from build123d import *

# Parameters (mm, degrees)
F0_W     = 93.609646
F0_H     = 82.611128
F1_DEPTH = 45.649247
F2_SIZE  = 1.27
F3_R     = 12.7


with BuildPart() as f1:
    # F0 (on Top) → F1 (new body)
    with BuildSketch(Plane.XY):
        with Locations((3.299557, -1.955293)):
            Rectangle(F0_W, F0_H)
    extrude(amount=F1_DEPTH)

    # F2
    f2_edges = [f1.edges().sort_by_distance(p)[0] for p in [
        (-43.505266, -43.260857, 22.824624),
        (50.10438, -43.260857, 22.824624),
        (3.299557, -43.260857, 0),
        (3.299557, -43.260857, 45.649247),
    ]]
    chamfer(f2_edges, length=F2_SIZE)

    # F3
    f3_edges = [f1.edges().sort_by_distance(p)[0] for p in [
        (50.10438, 39.350271, 22.824624),
        (-43.505266, 39.350271, 22.824624),
        (3.299557, 39.350271, 0),
        (3.299557, 39.350271, 45.649247),
    ]]
    fillet(f3_edges, radius=F3_R)


solid = f1.part
Could you check a few things on this model? Use its own coordinates, in mm. Give positions to 0.01 mm unless a question says otherwise; leave off trailing zeros. Write each loop counter-clockwise with the first axis right and the second up, starting at its lowest first coordinate (ties: lowest second). Pieces come first, ordered by that corner, then holes. Notation, with made-up numbers: (50, 82.5) -> (71, 82.5) arc R27 cw to (71, 113.5) -> close; hole circle Ø3 at (-39, -18.75). An arc over 180 degrees is marked (long way). Answer as a JSON object with one key per item and string values.
Q1. Suppose I cut it at C-C on y = 31. Write out the boundary of the cut face in (x, z), then the cut area to 3 significant figures.
Taken from the geometry:
{"outline": "(-42.74, 0.77) -> (49.34, 0.77) -> (49.34, 44.88) -> (-42.74, 44.88) -> close", "area": "4,060 mm²"}
Q2. Suppose I cut it at B-B on z = 3.5. Write out the boundary of the cut face in (x, y).
Taken from the geometry:
{"outline": "(-43.51, -41.99) -> (-42.24, -43.26) -> (48.83, -43.26) -> (50.1, -41.99) -> (50.1, 26.65) arc R12.7 ccw to (46.6, 35.41) -> (-40.01, 35.41) arc R12.7 ccw to (-43.51, 26.65) -> close"}
Q3. Please list where these lines run through material, in increasing order: L1, parallel to Y at x = -7.5, z = 6; L2, parallel to Y at x = -31, z = 29; L3, parallel to X at y = 28.5, z = 17.
Taken from the geometry:
{"L1": "y = -43.26 to 37.44", "L2": "y = -43.26 to 39.35", "L3": "x = -43.37 to 49.97"}
Q4. Suppose I cut it at A-A on x = 21. Write out the boundary of the cut face in (y, z), then the cut area to 3 significant figures.
Taken from the geometry:
{"outline": "(-43.26, 1.27) -> (-41.99, 0) -> (26.65, 0) arc R12.7 ccw to (39.35, 12.7) -> (39.35, 32.95) arc R12.7 ccw to (26.65, 45.65) -> (-41.99, 45.65) -> (-43.26, 44.38) -> close", "area": "3,700 mm²"}
